from build123d import *

# Parameters (mm, degrees)
SKETCH_1_W                       = 17.2
SKETCH_1_H                       = 19.6
EXTRUDE_1_DEPTH                  = 14.6
SKETCH_2_R                       = 9
EXTRUDE_2_DEPTH                  = 1
SKETCH_3_R                       = 6
EXTRUDE_3_DEPTH                  = 11.8
SKETCH_4_R                       = 4
EXTRUDE_4_DEPTH                  = 5
SKETCH_5_R                       = 5
EXTRUDE_5_DEPTH                  = 5.2
SKETCH_6_W                       = 0.8
SKETCH_6_H                       = 2
EXTRUDE_6_DEPTH                  = 4.5
PATTERN_LINEAR_1_COUNT           = 2
PATTERN_LINEAR_1_PITCH           = 5.3
PATTERN_LINEAR_2_COUNT           = 2
PATTERN_LINEAR_2_PITCH           = 4.7
PATTERN_LINEAR_2_COPY_1_SKETCH_W = 0.8
PATTERN_LINEAR_2_COPY_1_SKETCH_H = 2
PATTERN_LINEAR_2_COPY_1_DEPTH    = 4.5
PATTERN_LINEAR_3_COUNT           = 2
PATTERN_LINEAR_3_PITCH           = 5.3
PATTERN_LINEAR_3_COPY_1_SKETCH_W = 0.8
PATTERN_LINEAR_3_COPY_1_SKETCH_H = 2
PATTERN_LINEAR_3_COPY_1_DEPTH    = 4.5
PATTERN_LINEAR_3_COPY_2_SKETCH_W = 0.8
PATTERN_LINEAR_3_COPY_2_SKETCH_H = 2
PATTERN_LINEAR_3_COPY_2_DEPTH    = 4.5
PATTERN_LINEAR_3_COPY_3_SKETCH_W = 0.8
PATTERN_LINEAR_3_COPY_3_SKETCH_H = 2
PATTERN_LINEAR_3_COPY_3_DEPTH    = 4.5
PATTERN_START                    = -6.3
PATTERN_LINEAR_4_OUTLINE_W       = 0.8
PATTERN_LINEAR_4_OUTLINE_H       = 4.5
PATTERN_LINEAR_4_DEPTH           = 2
PATTERN_START_2                  = -1
PATTERN_LINEAR_4_2_OUTLINE_W     = 0.8
PATTERN_LINEAR_4_2_OUTLINE_H     = 4.5
PATTERN_LINEAR_4_2_DEPTH         = 2
PATTERN_START_3                  = 4.3
PATTERN_LINEAR_4_3_OUTLINE_W     = 0.8
PATTERN_LINEAR_4_3_OUTLINE_H     = 4.5
PATTERN_LINEAR_4_3_DEPTH         = 2
CUT_EXTRUDE_1_DEPTH              = 42.335335973


# Read off the part's stored shape, not the designer's step: 阵列(线性)4
with BuildPart() as part:
    # 草图1 → 凸台-拉伸1 (new body)
    with BuildSketch(Plane(origin=(0, 0, 0), x_dir=(1, 0, 0), z_dir=(0, 1, 0))):
        Rectangle(SKETCH_1_W, SKETCH_1_H)
    extrude(amount=EXTRUDE_1_DEPTH)

    # 草图2 → 凸台-拉伸2 (add)
    with BuildSketch(Plane(origin=(0, 14.6, 0), x_dir=(1, 0, 0), z_dir=(0, 1, 0))):
        with Locations(Location((0, 0, 0), (0, 0, 17.146209999))):
            Circle(SKETCH_2_R)
    extrude(amount=EXTRUDE_2_DEPTH)

    # 草图3 → 凸台-拉伸3 (add)
    with BuildSketch(Plane(origin=(0, 15.6, 0), x_dir=(1, 0, 0), z_dir=(0, 1, 0))):
        with Locations(Location((0, 0, 0), (0, 0, 270))):
            Circle(SKETCH_3_R)
    extrude(amount=EXTRUDE_3_DEPTH)

    # 草图4 → 凸台-拉伸4 (add)
    with BuildSketch(Plane(origin=(0, 27.4, 0), x_dir=(1, 0, 0), z_dir=(0, 1, 0))):
        with Locations(Location((0, 0, 0), (0, 0, 270))):
            Circle(SKETCH_4_R)
    extrude(amount=EXTRUDE_4_DEPTH)

    # 草图5 → 凸台-拉伸5 (add)
    with BuildSketch(Plane(origin=(0, 32.4, 0), x_dir=(1, 0, 0), z_dir=(0, 1, 0))):
        with Locations(Location((0, 0, 0), (0, 0, 270))):
            Circle(SKETCH_5_R)
    extrude(amount=EXTRUDE_5_DEPTH)

    # 草图6 → 凸台-拉伸6 (add)
    with BuildSketch(Plane.XZ):
        Rectangle(SKETCH_6_W, SKETCH_6_H)
    extrude_6 = extrude(amount=EXTRUDE_6_DEPTH)

    # 阵列(线性)1: 凸台-拉伸6 ×2
    with Locations(*[(0, 0, i * PATTERN_LINEAR_1_PITCH) for i in range(1, PATTERN_LINEAR_1_COUNT)]):
        add(extrude_6)

    # 阵列(线性)2: 凸台-拉伸6 ×2
    with Locations(*[(-i * PATTERN_LINEAR_2_PITCH, 0, 0) for i in range(1, PATTERN_LINEAR_2_COUNT)]):
        add(extrude_6)

    # 阵列(线性)2 copy 1 sketch → 阵列(线性)2 copy 1 (add)
    with BuildSketch(Plane(origin=(-4.7, 0, 5.3), x_dir=(1, 0, 0), z_dir=(0, -1, 0))):
        Rectangle(PATTERN_LINEAR_2_COPY_1_SKETCH_W, PATTERN_LINEAR_2_COPY_1_SKETCH_H)
    extrude(amount=PATTERN_LINEAR_2_COPY_1_DEPTH)

    # 阵列(线性)3: 凸台-拉伸6 ×2
    with Locations(*[(0, 0, -i * PATTERN_LINEAR_3_PITCH) for i in range(1, PATTERN_LINEAR_3_COUNT)]):
        add(extrude_6)

    # 阵列(线性)3 copy 1 sketch → 阵列(线性)3 copy 1 (add)
    with BuildSketch(Plane.XZ):
        Rectangle(PATTERN_LINEAR_3_COPY_1_SKETCH_W, PATTERN_LINEAR_3_COPY_1_SKETCH_H)
    extrude(amount=PATTERN_LINEAR_3_COPY_1_DEPTH)

    # 阵列(线性)3 copy 2 sketch → 阵列(线性)3 copy 2 (add)
    with BuildSketch(Plane(origin=(-4.7, 0, -5.3), x_dir=(1, 0, 0), z_dir=(0, -1, 0))):
        Rectangle(PATTERN_LINEAR_3_COPY_2_SKETCH_W, PATTERN_LINEAR_3_COPY_2_SKETCH_H)
    extrude(amount=PATTERN_LINEAR_3_COPY_2_DEPTH)

    # 阵列(线性)3 copy 3 sketch → 阵列(线性)3 copy 3 (add)
    with BuildSketch(Plane(origin=(-4.7, 0, 0), x_dir=(1, 0, 0), z_dir=(0, -1, 0))):
        Rectangle(PATTERN_LINEAR_3_COPY_3_SKETCH_W, PATTERN_LINEAR_3_COPY_3_SKETCH_H)
    extrude(amount=PATTERN_LINEAR_3_COPY_3_DEPTH)

    # 阵列(线性)4 outline → 阵列(线性)4 (add)
    with BuildSketch(Plane.XY.offset(PATTERN_START)):
        with Locations((4.7, -2.25)):
            Rectangle(PATTERN_LINEAR_4_OUTLINE_W, PATTERN_LINEAR_4_OUTLINE_H)
    extrude(amount=PATTERN_LINEAR_4_DEPTH)

    # Pattern Linear 4 2 outline → Pattern Linear 4 2 (add)
    with BuildSketch(Plane.XY.offset(PATTERN_START_2)):
        with Locations((4.7, -2.25)):
            Rectangle(PATTERN_LINEAR_4_2_OUTLINE_W, PATTERN_LINEAR_4_2_OUTLINE_H)
    extrude(amount=PATTERN_LINEAR_4_2_DEPTH)

    # Pattern Linear 4 3 outline → Pattern Linear 4 3 (add)
    with BuildSketch(Plane.XY.offset(PATTERN_START_3)):
        with Locations((4.7, -2.25)):
            Rectangle(PATTERN_LINEAR_4_3_OUTLINE_W, PATTERN_LINEAR_4_3_OUTLINE_H)
    extrude(amount=PATTERN_LINEAR_4_3_DEPTH)

    # 草图7 → 切除-拉伸1 (cut, through all)
    with BuildSketch(Plane.ZY.offset(5.1)):
        with BuildLine():
            Line((-0.642660902, -3.529284683), (-0.642660902, -1.428383643))
            ThreePointArc((-0.642660902, -1.428383643), (0.015637107, -0.770085634), (0.673935116, -1.428383643))
            Line((0.673935116, -1.428383643), (0.673935116, -3.529284683))
            ThreePointArc((0.673935116, -3.529284683), (0.015637107, -4.187582692), (-0.642660902, -3.529284683))
        make_face()
        with BuildLine():
            Line((-5.929653449, -3.387727592), (-5.841132285, -1.107614892))
            ThreePointArc((-5.841132285, -1.107614892), (-5.239978984, -0.551394487), (-4.683758579, -1.152547788))
            Line((-4.683758579, -1.152547788), (-4.772279743, -3.432660488))
            ThreePointArc((-4.772279743, -3.432660488), (-5.373433044, -3.988880894), (-5.929653449, -3.387727592))
        make_face()
        with BuildLine():
            Line((4.773595849, -3.425492164), (4.773595849, -1.220322784))
            ThreePointArc((4.773595849, -1.220322784), (5.285264786, -0.708653848), (5.796933722, -1.220322784))
            Line((5.796933722, -1.220322784), (5.796933722, -3.425492164))
            ThreePointArc((5.796933722, -3.425492164), (5.285264786, -3.937161101), (4.773595849, -3.425492164))
        make_face()
    extrude(amount=-CUT_EXTRUDE_1_DEPTH, mode=Mode.SUBTRACT)


solid = part.part
The model under review builds one solid part; all positions refer to its coordinate system, in mm. A direction names the side the tool comes from. Round coordinates to 2 decimals unless told otherwise and drop trailing zeros. Order: outer loops, then holes, each group sorted by start corner. A loop starts at its lowest first (then second) coordinate and runs counter-clockwise, first axis right, second up. Notation, with made-up numbers: (-8, 39.5) -> (43, 39.5) arc R35 ccw to (43, 78.5) -> close; hole circle Ø9 at (17, -26). An arc over 180 degrees is marked (long way). Write item = value, one per line. Start each with the question number.
Item 1: Consider section A-A on z = 8.25. Write out the cut boundary in (x, y).
Item 2: Consider section C-C on x = 0. Count the separate pieces of the cut face and the enclosed holes in it, plus the area to 3 significant figures.
Item 3: For line 1 along Y through (x, z) = (-4.75, -1.25); line 2 along X through (y, z) = (26.5, 0); line 3 along X through (y, z) = (34, -3), list the stretches that pass through material, from the lowest coordinate up.
Item 4: Clearance check with flat-ended pins moving along their axes: pin 1 Ø1 at (x, y) = (4.5, 18) entering from +Z; pin 2 Ø0.6 at (y, z) = (-3, -5) entering from -X; pin 3 Ø5.5 at (x, z) = (3, -7) entering from +Y; pin 4 Ø1 at (y, z) = (-2, -0.5) entering from +X. State where each tip first meets the part, or that it passes through.
Item 5: Consider section B-B on y = 13.5. Write out the cut boundary in (x, z).
Item 6: For faces 1 (the face through (-4.7, -2.2, -4.3)), 2 (the face through (1.802, 21.417, 5.723)), 3 (the face through (-5.1, -2, 6)), 4 (the face through (4.69, -3.99, -5.36)), list the 3-axis set-ups (+Z, -Z, +X, -X, +Y, -Y) from which the entire face can be reached by the end or side of a thin tool; tool diameter is ignored.
Conclusion:
q1.outline = (-8.6, 0) -> (8.6, 0) -> (8.6, 14.6) -> (3.6, 14.6) -> (3.6, 15.6) -> (-3.6, 15.6) -> (-3.6, 14.6) -> (-8.6, 14.6) -> close
q2.separate_pieces = 1
q2.enclosed_holes = 3
q2.area = 554 mm2
q3.line_1 = 0 to 27.4, 32.4 to 37.6
q3.line_2 = -6 to 6
q3.line_3 = -4 to 4
q4.pin_1 = 4.47
q4.pin_2 = -5.1
q4.pin_3 = 37.6
q4.pin_4 = 5.1
q5.outline = (-8.6, -9.8) -> (8.6, -9.8) -> (8.6, 9.8) -> (-8.6, 9.8) -> close
q6.face_1 = +X, -X, -Y
q6.face_2 = +Y
q6.face_3 = +Z, -Z, -X, -Y
q6.face_4 = +X, -X
